Input: part model. Units: mm. Frame: model coordinates. Give positions to 0.01 mm unless a question says otherwise; leave off trailing zeros. Loops run counter-clockwise (first coordinate to the right, second up) from the corner with the lowest first, then second, coordinate; pieces in that order, holes last. Notation, with made-up numbers: (-5.5, 28) - (36.5, 28) arc R17 cw to (36.5, 50) - close; hole circle Ø7 at (-30.5, 21). An arc over 180 degrees is marked (long way). Answer as a JSON object with one key per item and string values. Group by question number.
(1) Section query B-B (y = 5). Return loops of the section in (x, z).
(2) Section query D-D (z = 2.5). Return loops of the section in (x, y), plus the area to 3 significant figures.
(3) Mould query, pull axis X, two halves, no side actions, for faces 1 (the cylindrical face through (3.292, 21.586, 2.265)), 2 (the flat face through (0, 12, 1)), 3 (the flat face through (10, 13, 0)). Classes: +X half, -X half, draft (parallel to the pull), parting line (faces both ways), or undercut.
(4) Section query A-A (z = 0.8). Return loops of the section in (x, y).
(5) Section query C-C (x = 3.5). Return loops of the section in (y, z).
(6) Material intervals for L1, parallel to Y at x = 4.5, z = 1.9; L2, parallel to X at y = 5, z = 2.55; L3, parallel to Y at x = 3.25, z = 2, sorted ascending.
(7) Pin query (flat end, axial travel): P1, Ø3, axis at x = 3.5, y = 20, coming from the +Z side. Return the tip coordinate at first contact, or that it passes through.
```python
from build123d import *

# Parameters (mm, degrees)
SKETCH_1_W                  = 20
SKETCH_1_H                  = 25
SKETCH_1_R                  = 1.6
EXTRUDE_1_DEPTH             = 3
FILLET_1_R                  = 1
HOLE_WIZARD_M3_1_AT_2_COUNT = 2
HOLE_WIZARD_M3_1_AT_2_PITCH = 15


with BuildPart() as part:
    # ｽｹｯﾁ1 → ﾎﾞｽ - 押し出し1 (new body)
    with BuildSketch(Plane.XY):
        with Locations((10, 12.5)):
            Rectangle(SKETCH_1_W, SKETCH_1_H)
        with Locations((3.5, 5)):
            Circle(SKETCH_1_R, mode=Mode.SUBTRACT)
        with Locations((3.5, 20)):
            Circle(SKETCH_1_R, mode=Mode.SUBTRACT)
    extrude(amount=EXTRUDE_1_DEPTH)

    # ﾌｨﾚｯﾄ1
    fillet_1_edges = [part.edges().sort_by_distance(p)[0] for p in [
        (0, 25, 1.5),
        (20, 25, 1.5),
        (20, 0, 1.5),
        (0, 0, 1.5),
    ]]
    fillet(fillet_1_edges, radius=FILLET_1_R)

    # ｽｹｯﾁ3 → M3 丸皿ねじ用皿穴1 (revolve, cut)
    with BuildSketch(Plane(origin=(3.5, 20, 0), x_dir=(0, 1, 0), z_dir=(1, 0, 0))):
        Polygon((0, 0), (0, 3), (1.55, 3), (1.55, 1.6), (3.15, 0), align=None)
    hole_wizard_m3_1 = revolve(axis=Axis((3.5, 20, -6.35), (0, 0, 1)), mode=Mode.SUBTRACT)

    # M3 丸皿ねじ用皿穴1 at 2: M3 丸皿ねじ用皿穴1 ×2
    with Locations(*[(0, -i * HOLE_WIZARD_M3_1_AT_2_PITCH, 0) for i in range(1, HOLE_WIZARD_M3_1_AT_2_COUNT)]):
        add(hole_wizard_m3_1, mode=Mode.SUBTRACT)


solid = part.part
```
Recorded:
{
 "1": {"outline": "(0, 0) - (0.35, 0) - (1.9, 1.55) - (1.9, 3) - (0, 3) - close; (5.1, 1.55) - (6.65, 0) - (20, 0) - (20, 3) - (5.1, 3) - close"},
 "2": {"outline": "(0, 1) arc R1 ccw to (1, 0) - (19, 0) arc R1 ccw to (20, 1) - (20, 24) arc R1 ccw to (19, 25) - (1, 25) arc R1 ccw to (0, 24) - close; hole circle Ø3.2 at (3.5, 5); hole circle Ø3.2 at (3.5, 20)", "area": "483 mm^2"},
 "3": {"face 1": "undercut", "face 2": "-X half", "face 3": "draft"},
 "4": {"outline": "(0, 1) arc R1 ccw to (1, 0) - (19, 0) arc R1 ccw to (20, 1) - (20, 24) arc R1 ccw to (19, 25) - (1, 25) arc R1 ccw to (0, 24) - close; hole circle Ø4.7 at (3.5, 5); hole circle Ø4.7 at (3.5, 20)"},
 "5": {"outline": "(0, 0) - (1.85, 0) - (3.4, 1.55) - (3.4, 3) - (0, 3) - close; (6.6, 1.55) - (8.15, 0) - (16.85, 0) - (18.4, 1.55) - (18.4, 3) - (6.6, 3) - close; (21.6, 1.55) - (23.15, 0) - (25, 0) - (25, 3) - (21.6, 3) - close"},
 "6": {"L1": "y = 0 to 3.75, 6.25 to 18.75, 21.25 to 25", "L2": "x = 0 to 1.9, 5.1 to 20", "L3": "y = 0 to 3.42, 6.58 to 18.42, 21.58 to 25"},
 "7": {"P1": "passes through"}
}
